For this review, take the finished solid that the model builds, in its own axes (mm). Face numbers are marked on the shaded views. A direction names the side the tool comes from. Give positions to 0.01 mm unless a question says otherwise; leave off trailing zeros. Loops run counter-clockwise (first coordinate to the right, second up) from the corner with the lowest first, then second, coordinate; pieces in that order, holes last. Notation, with made-up numbers: (30.5, 73) - (37.5, 73) arc R18 ccw to (37.5, 92) - close; hole circle Ø1 at (-2, -36.75). An arc over 180 degrees is marked (long way). Put each result on its own line as item: value. Start each with the question number.
from build123d import *

# Parameters (mm, degrees)
BOSS_EXTRUDE1_DEPTH             = 11.5
SKETCH2_W                       = 8
SKETCH2_H                       = 6
BOSS_EXTRUDE2_DEPTH             = 8
CBORE_FOR_M2_5_SHCS1_AT_2_COUNT = 2
CBORE_FOR_M2_5_SHCS1_AT_2_PITCH = 26.100201416
FILLET2_R                       = 2


with BuildPart() as part:
    # Sketch1 → Boss-Extrude1 (new body)
    with BuildSketch(Plane.XY):
        Polygon((-9.05, 0), (-6.05, 0), (-6.05, 10.1), (6.05, 10.1), (6.05, 0), (9.05, 0), (9.05, 13.1), (-9.05, 13.1), align=None)
    extrude(amount=BOSS_EXTRUDE1_DEPTH)

    # Sketch2 → Boss-Extrude2 (add)
    with BuildSketch(Plane.XY.offset(11.5)):
        with Locations((-13.05, 3)):
            Rectangle(SKETCH2_W, SKETCH2_H)
        with Locations((13.05, 3)):
            Rectangle(SKETCH2_W, SKETCH2_H)
    extrude(amount=-BOSS_EXTRUDE2_DEPTH)

    # Sketch4 → CBORE for M2.5 SHCS1 (revolve, cut)
    with BuildSketch(Plane(origin=(-13.05, 6, 7.5), x_dir=(0, 0, 1), z_dir=(1, 0, 0))):
        Polygon((0, 0), (0, 6), (1.45, 6), (1.45, 2.5), (2.75, 2.5), (2.75, 0.025), (2.775, 0), align=None)
    cbore_for_m2_5_shcs1 = revolve(axis=Axis((-13.05, 12.35, 7.5), (0, -1, 0)), mode=Mode.SUBTRACT)

    # CBORE for M2.5 SHCS1 at 2: CBORE for M2.5 SHCS1 ×2
    with Locations(*[Vector(0.999992282957316, 0, 0.003928616272342698) * (i * CBORE_FOR_M2_5_SHCS1_AT_2_PITCH) for i in range(1, CBORE_FOR_M2_5_SHCS1_AT_2_COUNT)]):
        add(cbore_for_m2_5_shcs1, mode=Mode.SUBTRACT)

    # Fillet2
    fillet2_edges = [part.edges().sort_by_distance(p)[0] for p in [
        (-9.05, 13.1, 5.75),
        (9.05, 13.1, 5.75),
        (6.05, 10.1, 5.75),
        (-6.05, 10.1, 5.75),
        (-9.05, 3, 3.5),
        (-17.05, 3, 3.5),
        (-17.05, 3, 11.5),
        (9.05, 3, 3.5),
        (17.05, 3, 3.5),
        (17.05, 3, 11.5),
    ]]
    fillet(fillet2_edges, radius=FILLET2_R)


solid = part.part
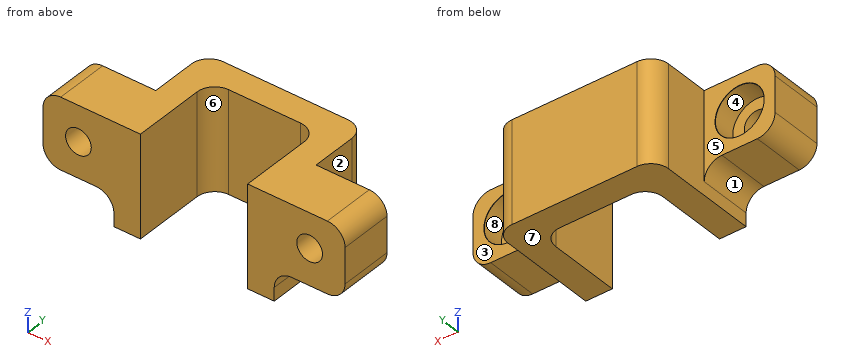
1) Mouldability with a two-part tool opening along X and no side actions: class the marked faces 1, 2, 3 and 4 as released by +X, released by -X, zero draft, split by the parting line, or undercut.
2) Wall thickness on probe 1 along X at (y, z) = (2.75, 7.5); probe 2 along X at (y, z) = (7.5, 1.25); probe 3 along X at (y, z) = (4.55, 7.5): over which ranges is each line inside the solid? List them lowest first.
3) Take a section at B-B on x = 13.05. State the section outline as (y, z) points (3 decimals).
4) Insertion check: P1, Ø4, axis at y = 9.5, z = 9.5, coming from the +X side; P2, Ø6.5, axis at x = -15, z = 6, coming from the +Y side; P3, Ø1.6, axis at x = 13, z = 7, coming from the +Y side; P4, Ø2.5, axis at x = 12.5, z = 8, coming from the +Y side. Each pin has a flat end and moves straight along its axis. Give the tip position at first contact, or say it passes through.
5) Take a section at C-C on y = 9.25. State the section outline as (x, z) points.
6) Take a section at D-D on z = 7.5. State how many separate pieces and enclosed holes the cut face has, and give its area (3 significant figures).
7) Machinability: for the marked faces 5, 6, 7 and 8, which of the approach directions +Z, -Z, +X, -X, +Y, -Y give a long, thin tool a straight path to every point of the face, cutting with its end or side? Answer none if there is none.
8) Take a section at A-A on y = 2.5. State the section outline as (x, z) points, and give its area (3 significant figures).
Answers follow:
1. face 1: released by -X
1. face 2: released by +X
1. face 3: zero draft
1. face 4: undercut
2. probe 1: -17.05 to -14.5, -11.6 to -6.05, 6.05 to 11.6, 14.5 to 17.05
2. probe 2: -9.05 to -6.05, 6.05 to 9.05
2. probe 3: -17.05 to -15.8, -10.3 to -6.05, 6.05 to 10.3, 15.8 to 17.05
3. outline: (0, 3.5) - (6, 3.5) - (6, 4.828) - (5.975, 4.853) - (3.5, 4.853) - (3.5, 6.153) - (0, 6.153) - close; (0, 9.053) - (3.5, 9.053) - (3.5, 10.353) - (5.975, 10.353) - (6, 10.378) - (6, 11.5) - (0, 11.5) - close
4. P1: x = 9.05
4. P2: y = 6
4. P3: through
4. P4: y = 3.5
5. outline: (-9.05, 0) - (-5.69, 0) - (-5.69, 11.5) - (-9.05, 11.5) - close; (5.69, 0) - (9.05, 0) - (9.05, 11.5) - (5.69, 11.5) - close
6. separate pieces: 3
6. enclosed holes: 0
6. area: 163 mm2
7. face 5: +Z, -Z, -X, +Y
7. face 6: +Z, -Z, -Y
7. face 7: -Z, +X, -X, +Y, -Y
7. face 8: +Y
8. outline: (-17.05, 5.5) arc R2 ccw to (-15.05, 3.5) - (-11.05, 3.5) arc R2 cw to (-9.05, 1.5) - (-9.05, 0) - (-6.05, 0) - (-6.05, 11.5) - (-15.05, 11.5) arc R2 ccw to (-17.05, 9.5) - close; (6.05, 0) - (9.05, 0) - (9.05, 1.5) arc R2 cw to (11.05, 3.5) - (15.05, 3.5) arc R2 ccw to (17.05, 5.5) - (17.05, 9.5) arc R2 ccw to (15.05, 11.5) - (6.05, 11.5) - close; hole circle Ø2.9 at (-13.05, 7.5); hole circle Ø2.9 at (13.05, 7.6)
8. area: 182 mm2
